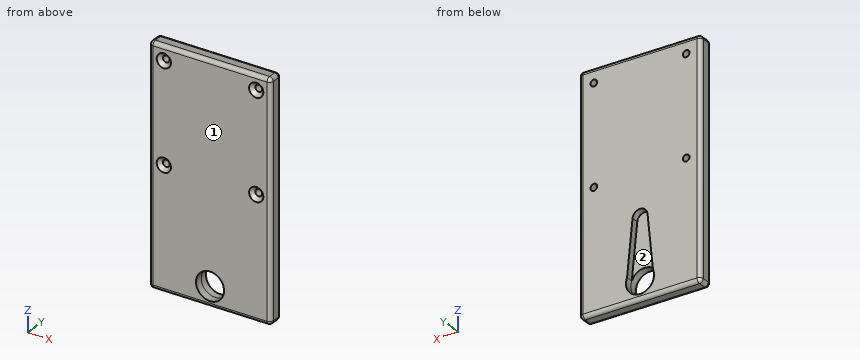
```python
from build123d import *

# Parameters (mm, degrees)
SKETCH1_W                     = 32.5
SKETCH1_H                     = 62.5
BASE_DEPTH                    = 4
SERVO_ARM_SLOT_DEPTH          = 1.9
SKETCH3_R                     = 3.75
SERVO_ARM_MOUNTING_HOLE_DEPTH = 65.612092521
SKETCH4_R                     = 0.9
SCANNER_MOUNTING_HOLES_DEPTH  = 65.701719452
MOUNTING_HOLE_CHAMFERS_SIZE   = 1
FILLET1_R                     = 1


with BuildPart() as part:
    # Sketch1 → Base (new body)
    with BuildSketch(Plane(origin=(0, 0, 0), x_dir=(1, 0, 0), z_dir=(0, 1, 0))):
        with Locations((0, 31.25)):
            Rectangle(SKETCH1_W, SKETCH1_H)
    extrude(amount=BASE_DEPTH)

    # Sketch2 → Servo Arm Slot (cut)
    with BuildSketch(Plane(origin=(0, 4, 0), x_dir=(1, 0, 0), z_dir=(0, 1, 0))):
        with BuildLine():
            Line((-3.46455, 55.814941361), (-2, 41.250001361))
            ThreePointArc((-2, 41.250001361), (0, 39.441022081), (2, 41.250001361))
            Line((2, 41.250001361), (3.46455, 55.814941361))
            ThreePointArc((3.46455, 55.814941361), (0, 61), (-3.46455, 55.814941361))
        make_face()
    extrude(amount=-SERVO_ARM_SLOT_DEPTH, mode=Mode.SUBTRACT)

    # Sketch3 → Servo Arm Mounting Hole (cut, through all)
    with BuildSketch(Plane(origin=(0, 2.1, 0), x_dir=(1, 0, 0), z_dir=(0, 1, 0))):
        with Locations(Location((0, 57.25, 0), (0, 0, 270))):
            Circle(SKETCH3_R)
    extrude(amount=-SERVO_ARM_MOUNTING_HOLE_DEPTH, mode=Mode.SUBTRACT)

    # Sketch4 → Scanner Mounting Holes (cut, through all)
    with BuildSketch(Plane.XZ):
        with Locations(Location((-12.35, -3.9, 0), (0, 0, 270))):
            Circle(SKETCH4_R)
        with Locations(Location((-12.35, -30.3, 0), (0, 0, 270))):
            Circle(SKETCH4_R)
        with Locations(Location((12.35, -30.3, 0), (0, 0, 90))):
            Circle(SKETCH4_R)
        with Locations(Location((12.35, -3.9, 0), (0, 0, 90))):
            Circle(SKETCH4_R)
    extrude(amount=-SCANNER_MOUNTING_HOLES_DEPTH, mode=Mode.SUBTRACT)

    # Mounting Hole Chamfers
    mounting_hole_chamfers_edges = [part.edges().sort_by_distance(p)[0] for p in [
        (12.35, 0, -4.8),
        (12.35, 0, -31.2),
        (-12.35, 0, -29.4),
        (-12.35, 0, -3),
    ]]
    chamfer(mounting_hole_chamfers_edges, length=MOUNTING_HOLE_CHAMFERS_SIZE)

    # Fillet1
    fillet1_edges = [part.edges().sort_by_distance(p)[0] for p in [
        (16.25, 4, -31.25),
        (0, 4, -62.5),
        (-16.25, 4, -31.25),
        (0, 0, -62.5),
        (16.25, 0, -31.25),
        (0, 0, 0),
        (-16.25, 0, -31.25),
        (-16.25, 2, -62.5),
        (16.25, 2, -62.5),
        (16.25, 2, 0),
        (-16.25, 2, 0),
        (0, 4, 0),
    ]]
    fillet(fillet1_edges, radius=FILLET1_R)


solid = part.part
```
Design review of the part built by this model. Coordinates are the model's own, in mm. Face numbers are marked on the shaded views. A direction names the side the tool comes from. Coordinates: 2 decimals unless noted, no trailing zeros. Order: outer loops, then holes, each group sorted by start corner. A loop starts at its lowest first (then second) coordinate and runs counter-clockwise, first axis right, second up.
1) Take a section at C-C, the plane x = -12.35. Give the boundary of the cut face in (y, z), and give its area (3 significant figures).
2) Take a section at D-D, the plane z = -56.5. Give the boundary of the cut face in (x, y), and give its area (3 significant figures).
3) Take a section at B-B, the plane z = -3.9. Give the boundary of the cut face in (x, y).
4) For the marked faces 1 and 2, list the 3-axis set-ups (+Z, -Z, +X, -X, +Y, -Y) from which the entire face can be reached by the end or side of a thin tool; tool diameter is ignored.
5) Take a section at A-A, the plane x = 0. Give the boundary of the cut face in (y, z), and give its area (3 significant figures).
6) Wall thickness on line 1 along X through (y, z) = (3.1, -3.9); line 2 along Z through (x, y) = (0, 1.15); line 3 along Z through (x, y) = (0, 3.05): over which ranges is each line inside the solid? List them lowest first.
Returned:
1. outline: (0, -61.5) arc R1 ccw to (1, -62.5) - (3, -62.5) arc R1 ccw to (4, -61.5) - (4, -31.2) - (1, -31.2) - (0, -32.2) - close; (0, -28.4) - (1, -29.4) - (4, -29.4) - (4, -4.8) - (1, -4.8) - (0, -5.8) - close; (0, -2) - (1, -3) - (4, -3) - (4, -1) arc R1 ccw to (3, 0) - (1, 0) arc R1 ccw to (0, -1) - close
1. area: 233 mm2
2. outline: (-16.25, 1) arc R1 ccw to (-15.25, 0) - (-3.67, 0) - (-3.67, 4) - (-15.25, 4) arc R1 ccw to (-16.25, 3) - close; (3.67, 0) - (15.25, 0) arc R1 ccw to (16.25, 1) - (16.25, 3) arc R1 ccw to (15.25, 4) - (3.67, 4) - close
2. area: 99.7 mm2
3. outline: (-16.25, 1) arc R1 ccw to (-15.25, 0) - (-14.25, 0) - (-13.25, 1) - (-13.25, 4) - (-15.25, 4) arc R1 ccw to (-16.25, 3) - close; (-11.45, 1) - (-10.45, 0) - (10.45, 0) - (11.45, 1) - (11.45, 4) - (-11.45, 4) - close; (13.25, 1) - (14.25, 0) - (15.25, 0) arc R1 ccw to (16.25, 1) - (16.25, 3) arc R1 ccw to (15.25, 4) - (13.25, 4) - close
4. face 1: +Z, -Z, +X, -X, -Y
4. face 2: +Y
5. outline: (0, -61.5) arc R1 ccw to (1, -62.5) - (3, -62.5) arc R1 ccw to (4, -61.5) - (4, -61) - (0, -61) - close; (0, -53.5) - (2.1, -53.5) - (2.1, -39.44) - (4, -39.44) - (4, -1) arc R1 ccw to (3, 0) - (1, 0) arc R1 ccw to (0, -1) - close
5. area: 192 mm2
6. line 1: x = -16.24 to -13.25, -11.45 to 11.45, 13.25 to 16.24
6. line 2: z = -62.5 to -61, -53.5 to 0
6. line 3: z = -62.5 to -61, -39.44 to 0
